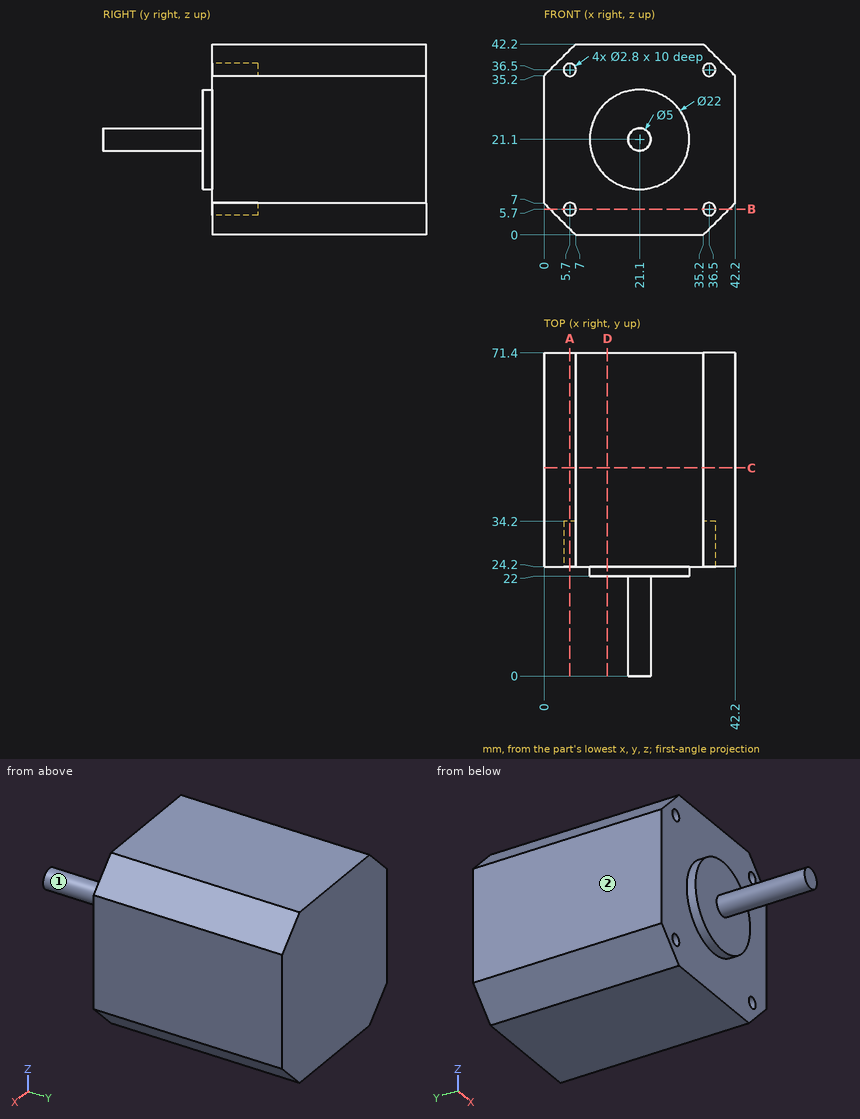
Geometry check sheet. Reference: drawing and pictorial views, mm from the part's lowest x, y, z. A direction names the side the tool comes from. Round coordinates to 2 decimals unless told otherwise and drop trailing zeros. Loops run counter-clockwise (first coordinate to the right, second up) from the corner with the lowest first, then second, coordinate; pieces in that order, holes last. Notation, with made-up numbers: (70, 47.25) - (123, 47.25) arc R34 cw to (123, 80.25) - close; hole circle Ø9 at (-32.75, 59.5). An arc over 180 degrees is marked (long way). Use a Markdown table: item, result. Add a question column.
1. Gauge pin test, flat ends, axial feed: pin 1 (3 mm diameter, centred on x = 35, z = 20.5, fed in from -Y); pin 2 (1.4 mm diameter, centred on x = 5.5, z = 36.5, fed in from -Y). Record the tip position at first contact, or that the pin passes through.
2. Section check A-A, the plane x = 5.7. Record the boundary of the cut face in (y, z), plus the area to 3 significant figures.
3. Section check D-D, the plane x = 14. Record the boundary of the cut face in (y, z).
4. Section check B-B, the plane z = 5.7. Record the boundary of the cut face in (x, y).
5. Thickness scan on probe 1 along Z at (x, y) = (36.5, 27.75); probe 2 along X at (y, z) = (29, 37.5); probe 3 along X at (y, z) = (31, 36). Record the ranges inside material, lowest first. Write a range as [from, to].
6. Section check C-C, the plane y = 46. Record the boundary of the cut face in (x, z), plus the area to 3 significant figures.
7. Access from +Z, -Z, +X, -X, +Y, -Y to the whole of each face (thin tool, end or side, straight path). Record for the marked faces 1 and 2.
Checks:
| question | item | result |
|---|---|---|
| 1 | pin 1 | stops at y = 24.2 |
| 1 | pin 2 | stops at y = 34.2 |
| 2 | outline | (24.2, 1.3) - (71.4, 1.3) - (71.4, 40.9) - (24.2, 40.9) - (24.2, 37.9) - (34.2, 37.9) - (34.2, 35.1) - (24.2, 35.1) - (24.2, 7.1) - (34.2, 7.1) - (34.2, 4.3) - (24.2, 4.3) - close |
| 2 | area | 1,810 mm^2 |
| 3 | outline | (22, 12.7) - (24.2, 12.7) - (24.2, 0) - (71.4, 0) - (71.4, 42.2) - (24.2, 42.2) - (24.2, 29.5) - (22, 29.5) - close |
| 4 | outline | (1.3, 24.2) - (4.3, 24.2) - (4.3, 34.2) - (7.1, 34.2) - (7.1, 24.2) - (35.1, 24.2) - (35.1, 34.2) - (37.9, 34.2) - (37.9, 24.2) - (40.9, 24.2) - (40.9, 71.4) - (1.3, 71.4) - close |
| 5 | probe 1 | z = [1.3, 4.3], [7.1, 35.1], [37.9, 40.9] |
| 5 | probe 2 | x = [2.3, 4.72], [6.68, 35.52], [37.48, 39.9] |
| 5 | probe 3 | x = [0.8, 4.39], [7.01, 35.19], [37.81, 41.4] |
| 6 | outline | (0, 7) - (7, 0) - (35.2, 0) - (42.2, 7) - (42.2, 35.2) - (35.2, 42.2) - (7, 42.2) - (0, 35.2) - close |
| 6 | area | 1,680 mm^2 |
| 7 | face 1 | -Y |
| 7 | face 2 | +Z, -Z, -X, +Y, -Y |
